Here's how the part is built. I have some questions about the finished solid (model axes, mm). Face numbers are marked on the shaded views. A direction names the side the tool comes from. Round coordinates to 2 decimals unless told otherwise and drop trailing zeros. Write each loop counter-clockwise with the first axis right and the second up, starting at its lowest first coordinate (ties: lowest second). Pieces come first, ordered by that corner, then holes. Notation, with made-up numbers: (-25.75, 9.5) - (14.25, 9.5) arc R21 cw to (14.25, 35.5) - close; hole circle Ø4 at (60.5, 16). An arc over 180 degrees is marked (long way). Use one line per item in the form item = value. Start each with the question number.
1. I want a section at C-C, the plane x = 11. List the corners of the cut face in (y, z) for me.
2. I want a section at B-B, the plane y = 4. List the corners of the cut face in (x, z) for me, plus the area to 3 significant figures.
3. If I drill on line 1 along X through (y, z) = (0.75, -9.75); line 2 along Z through (x, y) = (7, 4.25); line 3 along Z through (x, y) = (13.25, 0.75), over which ranges is the centre line in solid material (lowest first)?
4. We'd pull the mould along Z, two halves only. Please class the marked faces 1, 2 and 3: +Z half, -Z half, draft (parallel to the pull), parting line (faces both ways), or undercut.
5. I want a section at A-A, the plane x = 3.5. List the corners of the cut face in (y, z) for me.
6. I want a section at D-D, the plane z = 0. List the corners of the cut face in (x, y) for me, plus the area to 3 significant figures.
7. Will these pins go through, and if not, where does the flat tip stop? pin 1 (1.5 mm diameter, centred on x = 24.5, y = 5, fed in from +Z); pin 2 (2.5 mm diameter, centred on x = 26.5, z = 10.37, fed in from -Y); pin 3 (1.6 mm diameter, centred on x = 9.5, z = -11, fed in from +Y); pin 4 (3 mm diameter, centred on x = 17.5, z = -0.5, fed in from -Y).
8. Which directions (+Z, -Z, +X, -X, +Y, -Y) give clear straight access to the entire face, cutting with the end or side of a thin tool? Please do the marked faces 4, 5 and 6.
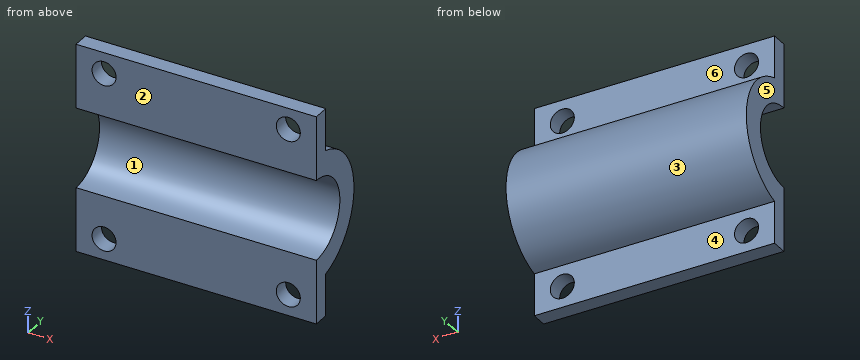
```python
from build123d import *

# Parameters (mm, degrees)
EXTRUDE_1_DEPTH     = 30
SKETCH_2_R          = 1.5
CUT_EXTRUDE_1_DEPTH = 10


with BuildPart() as part:
    # 草图1 → 凸台-拉伸1 (new body)
    with BuildSketch(Plane(origin=(0, 0, 0), x_dir=(0, 0, -1), z_dir=(1, 0, 0))):
        with BuildLine():
            Line((-5, 0), (-13, 0))
            Line((-13, 0), (-13, 2))
            Line((-13, 2), (-7.745966692, 2))
            ThreePointArc((-7.745966692, 2), (0, 8), (7.745966692, 2))
            Line((7.745966692, 2), (13, 2))
            Line((13, 2), (13, 0))
            Line((13, 0), (5, 0))
            ThreePointArc((5, 0), (0, 5), (-5, 0))
        make_face()
    extrude(amount=EXTRUDE_1_DEPTH)

    # 草图2 → 切除-拉伸1 (cut)
    with BuildSketch(Plane.XZ):
        with Locations(Location((26.5, -10.372983346, 0), (0, 0, 270))):
            Circle(SKETCH_2_R)
        with Locations(Location((3.5, -10.372983346, 0), (0, 0, 270))):
            Circle(SKETCH_2_R)
        with Locations(Location((3.5, 10.372983346, 0), (0, 0, 270))):
            Circle(SKETCH_2_R)
        with Locations(Location((26.5, 10.372983346, 0), (0, 0, 270))):
            Circle(SKETCH_2_R)
    extrude(amount=-CUT_EXTRUDE_1_DEPTH, mode=Mode.SUBTRACT)


solid = part.part
```
Model answer:
q1.outline = (0, -13) - (2, -13) - (2, -7.75) arc R8 ccw to (2, 7.75) - (2, 13) - (0, 13) - (0, 5) arc R5 cw to (0, -5) - close
q2.outline = (0, -6.93) - (30, -6.93) - (30, -3) - (0, -3) - close; (0, 3) - (30, 3) - (30, 6.93) - (0, 6.93) - close
q2.area = 236 mm2
q3.line_1 = 0 to 2.14, 4.86 to 25.14, 27.86 to 30
q3.line_2 = -6.78 to -2.63, 2.63 to 6.78
q3.line_3 = -13 to -4.94, 4.94 to 13
q4.face_1 = undercut
q4.face_2 = draft
q4.face_3 = parting line
q5.outline = (0, -13) - (2, -13) - (2, -11.87) - (0, -11.87) - close; (0, -8.87) - (2, -8.87) - (2, -7.75) arc R8 ccw to (2, 7.75) - (2, 8.87) - (0, 8.87) - (0, 5) arc R5 cw to (0, -5) - close; (0, 11.87) - (2, 11.87) - (2, 13) - (0, 13) - close
q6.outline = (0, 5) - (30, 5) - (30, 8) - (0, 8) - close
q6.area = 90.0 mm2
q7.pin_1 = 6.78
q7.pin_2 = through
q7.pin_3 = 2
q7.pin_4 = 4.58
q8.face_4 = -Z, +X, -X, +Y
q8.face_5 = +Z, -Z, -X, +Y, -Y
q8.face_6 = +Z, +X, -X, +Y
